from build123d import *

# Parameters (mm, degrees)
BASE_FLANGE1_DEPTH = 120
CUT_EXTRUDE1_REACH = 126.76
SKETCH6_R          = 3
LPATTERN1_COUNT    = 2
LPATTERN1_PITCH    = 40
FILLET1_R          = 3
CUT_EXTRUDE2_REACH = 126.76
SKETCH7_R          = 3


# Sheet-metal steps are written as plain solids
with BuildPart() as part:
    # Sketch1 → Base-Flange1 (new body)
    with BuildSketch(Plane(origin=(0, 0, 0), x_dir=(1, 0, 0), z_dir=(0, 1, 0))):
        with BuildLine():
            Line((-26, -18), (-26, -1))
            ThreePointArc((-26, -1), (-25.707106781, -0.292893219), (-25, 0))
            Line((-25, 0), (25, 0))
            ThreePointArc((25, 0), (25.707106781, -0.292893219), (26, -1))
            Line((26, -1), (26, -18))
            Line((26, -18), (29, -18))
            Line((29, -18), (29, -1))
            ThreePointArc((29, -1), (27.828427125, 1.828427125), (25, 3))
            Line((25, 3), (-25, 3))
            ThreePointArc((-25, 3), (-27.828427125, 1.828427125), (-29, -1))
            Line((-29, -1), (-29, -18))
            Line((-29, -18), (-26, -18))
        make_face()
    extrude(amount=BASE_FLANGE1_DEPTH)

    # Sketch6 → Cut-Extrude1 (cut, up to next)
    with BuildSketch(Plane.XY, mode=Mode.PRIVATE) as cut_extrude1_sk1:
        with Locations((-17.2, 8)):
            Circle(SKETCH6_R)
    cut_extrude1_tool1 = extrude(cut_extrude1_sk1.sketch, amount=-CUT_EXTRUDE1_REACH, mode=Mode.PRIVATE) & part.part
    # Sketch6 → Cut-Extrude1 (cut, up to next)
    with BuildSketch(Plane.XY, mode=Mode.PRIVATE) as cut_extrude1_sk2:
        with Locations((17.2, 8)):
            Circle(SKETCH6_R)
    cut_extrude1_tool2 = extrude(cut_extrude1_sk2.sketch, amount=-CUT_EXTRUDE1_REACH, mode=Mode.PRIVATE) & part.part
    # Sketch6 → Cut-Extrude1 (cut, up to next)
    with BuildSketch(Plane.XY, mode=Mode.PRIVATE) as cut_extrude1_sk3:
        with BuildLine():
            Line((-11.9, 22.5), (-11.9, 17.5))
            ThreePointArc((-11.9, 17.5), (-12.9, 16.5), (-13.9, 17.5))
            Line((-13.9, 17.5), (-13.9, 22.5))
            ThreePointArc((-13.9, 22.5), (-12.9, 23.5), (-11.9, 22.5))
        make_face()
    cut_extrude1_tool3 = extrude(cut_extrude1_sk3.sketch, amount=-CUT_EXTRUDE1_REACH, mode=Mode.PRIVATE) & part.part
    # Sketch6 → Cut-Extrude1 (cut, up to next)
    with BuildSketch(Plane.XY, mode=Mode.PRIVATE) as cut_extrude1_sk4:
        with BuildLine():
            Line((-22.5, 22.5), (-22.5, 17.5))
            ThreePointArc((-22.5, 17.5), (-21.5, 16.5), (-20.5, 17.5))
            Line((-20.5, 17.5), (-20.5, 22.5))
            ThreePointArc((-20.5, 22.5), (-21.5, 23.5), (-22.5, 22.5))
        make_face()
    cut_extrude1_tool4 = extrude(cut_extrude1_sk4.sketch, amount=-CUT_EXTRUDE1_REACH, mode=Mode.PRIVATE) & part.part
    # Sketch6 → Cut-Extrude1 (cut, up to next)
    with BuildSketch(Plane.XY, mode=Mode.PRIVATE) as cut_extrude1_sk5:
        with BuildLine():
            Line((5.3, 22.5), (5.3, 17.5))
            ThreePointArc((5.3, 17.5), (4.3, 16.5), (3.3, 17.5))
            Line((3.3, 17.5), (3.3, 22.5))
            ThreePointArc((3.3, 22.5), (4.3, 23.5), (5.3, 22.5))
        make_face()
    cut_extrude1_tool5 = extrude(cut_extrude1_sk5.sketch, amount=-CUT_EXTRUDE1_REACH, mode=Mode.PRIVATE) & part.part
    # Sketch6 → Cut-Extrude1 (cut, up to next)
    with BuildSketch(Plane.XY, mode=Mode.PRIVATE) as cut_extrude1_sk6:
        with BuildLine():
            Line((-5.3, 22.5), (-5.3, 17.5))
            ThreePointArc((-5.3, 17.5), (-4.3, 16.5), (-3.3, 17.5))
            Line((-3.3, 17.5), (-3.3, 22.5))
            ThreePointArc((-3.3, 22.5), (-4.3, 23.5), (-5.3, 22.5))
        make_face()
    cut_extrude1_tool6 = extrude(cut_extrude1_sk6.sketch, amount=-CUT_EXTRUDE1_REACH, mode=Mode.PRIVATE) & part.part
    # Sketch6 → Cut-Extrude1 (cut, up to next)
    with BuildSketch(Plane.XY, mode=Mode.PRIVATE) as cut_extrude1_sk7:
        with BuildLine():
            Line((22.5, 22.5), (22.5, 17.5))
            ThreePointArc((22.5, 17.5), (21.5, 16.5), (20.5, 17.5))
            Line((20.5, 17.5), (20.5, 22.5))
            ThreePointArc((20.5, 22.5), (21.5, 23.5), (22.5, 22.5))
        make_face()
    cut_extrude1_tool7 = extrude(cut_extrude1_sk7.sketch, amount=-CUT_EXTRUDE1_REACH, mode=Mode.PRIVATE) & part.part
    # Sketch6 → Cut-Extrude1 (cut, up to next)
    with BuildSketch(Plane.XY, mode=Mode.PRIVATE) as cut_extrude1_sk8:
        with BuildLine():
            Line((11.9, 22.5), (11.9, 17.5))
            ThreePointArc((11.9, 17.5), (12.9, 16.5), (13.9, 17.5))
            Line((13.9, 17.5), (13.9, 22.5))
            ThreePointArc((13.9, 22.5), (12.9, 23.5), (11.9, 22.5))
        make_face()
    cut_extrude1_tool8 = extrude(cut_extrude1_sk8.sketch, amount=-CUT_EXTRUDE1_REACH, mode=Mode.PRIVATE) & part.part
    cut_extrude1_1 = cut_extrude1_tool1.solids().sort_by_distance((-17.2, 8, 0))[0]
    add(cut_extrude1_1, mode=Mode.SUBTRACT)
    cut_extrude1_2 = cut_extrude1_tool2.solids().sort_by_distance((17.2, 8, 0))[0]
    add(cut_extrude1_2, mode=Mode.SUBTRACT)
    cut_extrude1_3 = cut_extrude1_tool3.solids().sort_by_distance((-12.9, 20, 0))[0]
    add(cut_extrude1_3, mode=Mode.SUBTRACT)
    cut_extrude1_4 = cut_extrude1_tool4.solids().sort_by_distance((-21.5, 20, 0))[0]
    add(cut_extrude1_4, mode=Mode.SUBTRACT)
    cut_extrude1_5 = cut_extrude1_tool5.solids().sort_by_distance((4.3, 20, 0))[0]
    add(cut_extrude1_5, mode=Mode.SUBTRACT)
    cut_extrude1_6 = cut_extrude1_tool6.solids().sort_by_distance((-4.3, 20, 0))[0]
    add(cut_extrude1_6, mode=Mode.SUBTRACT)
    cut_extrude1_7 = cut_extrude1_tool7.solids().sort_by_distance((21.5, 20, 0))[0]
    add(cut_extrude1_7, mode=Mode.SUBTRACT)
    cut_extrude1_8 = cut_extrude1_tool8.solids().sort_by_distance((12.9, 20, 0))[0]
    add(cut_extrude1_8, mode=Mode.SUBTRACT)
    cut_extrude1 = cut_extrude1_1 + cut_extrude1_2 + cut_extrude1_3 + cut_extrude1_4 + cut_extrude1_5 + cut_extrude1_6 + cut_extrude1_7 + cut_extrude1_8  # Cut-Extrude1 as one shape, for the pattern or mirror that repeats it

    # LPattern1: Cut-Extrude1 ×2
    with Locations(*[(0, i * LPATTERN1_PITCH, 0) for i in range(1, LPATTERN1_COUNT)]):
        add(cut_extrude1, mode=Mode.SUBTRACT)

    # Fillet1
    fillet1_edges = [part.edges().sort_by_distance(p)[0] for p in [
        (27.5, 0, 18),
        (-27.5, 0, 18),
        (27.5, 120, 18),
        (-27.5, 120, 18),
    ]]
    fillet(fillet1_edges, radius=FILLET1_R)

    # Sketch7 → Cut-Extrude2 (cut, up to next)
    with BuildSketch(Plane.XY, mode=Mode.PRIVATE) as cut_extrude2_sk1:
        with Locations((0, 114)):
            Circle(SKETCH7_R)
    cut_extrude2_tool1 = extrude(cut_extrude2_sk1.sketch, amount=-CUT_EXTRUDE2_REACH, mode=Mode.PRIVATE) & part.part
    # Sketch7 → Cut-Extrude2 (cut, up to next)
    with BuildSketch(Plane.XY, mode=Mode.PRIVATE) as cut_extrude2_sk2:
        with Locations((-15, 102)):
            Circle(SKETCH7_R)
    cut_extrude2_tool2 = extrude(cut_extrude2_sk2.sketch, amount=-CUT_EXTRUDE2_REACH, mode=Mode.PRIVATE) & part.part
    # Sketch7 → Cut-Extrude2 (cut, up to next)
    with BuildSketch(Plane.XY, mode=Mode.PRIVATE) as cut_extrude2_sk3:
        with Locations((15, 102)):
            Circle(SKETCH7_R)
    cut_extrude2_tool3 = extrude(cut_extrude2_sk3.sketch, amount=-CUT_EXTRUDE2_REACH, mode=Mode.PRIVATE) & part.part
    add(cut_extrude2_tool1.solids().sort_by_distance((0, 114, 0))[0], mode=Mode.SUBTRACT)
    add(cut_extrude2_tool2.solids().sort_by_distance((-15, 102, 0))[0], mode=Mode.SUBTRACT)
    add(cut_extrude2_tool3.solids().sort_by_distance((15, 102, 0))[0], mode=Mode.SUBTRACT)


solid = part.part
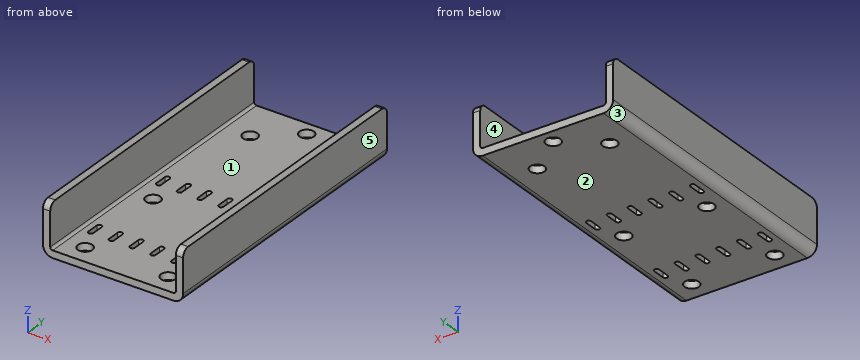
Work out the finished part from the listing and answer in its coordinate system (mm). Face numbers are marked on the shaded views. A direction names the side the tool comes from. Coordinates: 2 decimals unless noted, no trailing zeros. Write each loop counter-clockwise with the first axis right and the second up, starting at its lowest first coordinate (ties: lowest second). Pieces come first, ordered by that corner, then holes. Notation, with made-up numbers: (1.5, 14) - (22.5, 14) arc R30 ccw to (22.5, 40) - close; hole circle Ø5 at (85.25, 23.5). An arc over 180 degrees is marked (long way). One line per question, with ' | ' between items.
1) Flat-ended cylindrical pins translate along their axes: P1, Ø10, axis at x = 13, y = 23, coming from the -Z side; P2, Ø0.9, axis at y = 21, z = -1, coming from the -X side; P3, Ø1.5, axis at y = 59, z = -2, coming from the +X side; P4, Ø2.5, axis at y = 20, z = -2, coming from the -X side. Find the tip coordinate at first contact, or state that the pin passes through.
Checks:
P1: z = -3 | P2: x = -28.69 | P3: x = 28.31 | P4: x = -28.6
2) Find section B-B, the plane y = 102. Determine the outline of the cut face in (x, z), and give its area (3 significant figures).
Checks:
outline: (-29, 1) arc R4 ccw to (-25, -3) - (-18, -3) - (-18, 0) - (-25, 0) arc R1 cw to (-26, 1) - (-26, 18) - (-29, 18) - close; (-12, -3) - (12, -3) - (12, 0) - (-12, 0) - close; (18, -3) - (25, -3) arc R4 ccw to (29, 1) - (29, 18) - (26, 18) - (26, 1) arc R1 cw to (25, 0) - (18, 0) - close | area: 240 mm2
3) Find section C-C, the plane z = 12. Determine the outline of the cut face in (x, y).
Checks:
outline: (-29, 0) - (-26, 0) - (-26, 120) - (-29, 120) - close; (26, 0) - (29, 0) - (29, 120) - (26, 120) - close
4) For the marked faces 4 and 5, determine the directions among +Z, -Z, +X, -X, +Y, -Y from which every point of the face is accessible in a straight line to the end or side of a thin tool.
Checks:
face 4: +Z, +Y, -Y | face 5: +Z, -Z, +X, +Y, -Y
5) Find section A-A, the plane x = 0. Determine the outline of the cut face in (y, z).
Checks:
outline: (0, -3) - (111, -3) - (111, 0) - (0, 0) - close; (117, -3) - (120, -3) - (120, 0) - (117, 0) - close
6) The mould has two halves that part along X. Classify the marked faces 1, 2 and 3: +X half, -X half, draft (parallel to the pull), parting line (faces both ways), or undercut.
Checks:
face 1: undercut | face 2: draft | face 3: -X half
7) Consider probe 1 along X at (y, z) = (66.5, 10); probe 2 along Y at (x, z) = (15, -0.7); probe 3 along Y at (x, z) = (-12.5, -1.25). Determine where each line is inside the solid, lowest interval first. Write a range as [from, to].
Checks:
probe 1: [-29, -26], [26, 29] | probe 2: [0, 5.96], [10.04, 45.96], [50.04, 99], [105, 120] | probe 3: [0, 16.58], [23.42, 56.58], [63.42, 100.34], [103.66, 120]
8) Find section D-D, the plane y = 65. Determine the outline of the cut face in (x, z).
Checks:
outline: (-29, 1) arc R4 ccw to (-25, -3) - (25, -3) arc R4 ccw to (29, 1) - (29, 18) - (26, 18) - (26, 1) arc R1 cw to (25, 0) - (-25, 0) arc R1 cw to (-26, 1) - (-26, 18) - (-29, 18) - close
